Read the model definition and answer for the solid it produces. Units are mm, in the model's axes. Face numbers are marked on the shaded views. A direction names the side the tool comes from. Give positions to 0.01 mm unless a question says otherwise; leave off trailing zeros. Loops run counter-clockwise (first coordinate to the right, second up) from the corner with the lowest first, then second, coordinate; pieces in that order, holes last.
(1) Find section B-B, the plane y = 15. Write down the section's boundary in (x, z).
(2) Which of the six approach directions +Z, -Z, +X, -X, +Y, -Y give full straight-line access (tool end or side, diameter ignored) to the marked faces 4, 5 and 6?
(3) Find section D-D, the plane x = -5. Write down the section's boundary in (y, z), then the cut area to 3 significant figures.
(4) Determine the mould class of the marked faces 1, 2 and 3 for opening direction X: pulls with the +X half, pulls with the -X half, needs draft (parallel to the pull), parting line crosses it, or undercut.
(5) Find section C-C, the plane z = 1.5. Write down the section's boundary in (x, y).
(6) Each of these flat-tipped pins is pushed along its axis until it touches: P1, Ø4.5, axis at x = 7.5, y = 15, coming from the +Z side; P2, Ø4, axis at y = 10.5, z = 3, coming from the -X side; P3, Ø4, axis at x = -5, z = 6, coming from the +Y side. Where does it stop, or does it pass through?
(7) Find section A-A, the plane x = 7.5. Write down the section's boundary in (y, z), then the cut area to 3 significant figures.
(8) Straight lines are drawn through the part: probe 1 along Y at (x, z) = (7.5, 2.5); probe 2 along X at (y, z) = (0.7, 0); probe 3 along Z at (x, y) = (-5, 4.1). For each, find the intervals that lie inside material, in ascending order.
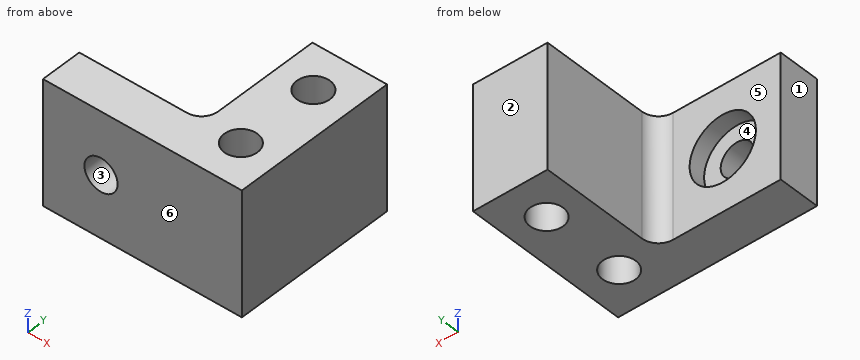
```python
from build123d import *

# Parameters (mm, degrees)
SKETCH1_W           = 24
SKETCH1_H           = 15
BOSS_EXTRUDE2_DEPTH = 5
SKETCH8_W           = 9
SKETCH8_H           = 15
BOSS_EXTRUDE3_DEPTH = 15
CUT_EXTRUDE3_REACH  = 7
SKETCH10_R          = 2
SKETCH9_R           = 4
CUT_EXTRUDE4_DEPTH  = 2
CUT_EXTRUDE5_REACH  = 17
SKETCH11_R          = 2
FILLET4_R           = 2


with BuildPart() as part:
    # Sketch1 → Boss-Extrude2 (new body)
    with BuildSketch(Plane(origin=(0, 0, 0), x_dir=(1, 0, 0), z_dir=(0, 1, 0))):
        Rectangle(SKETCH1_W, SKETCH1_H)
    extrude(amount=BOSS_EXTRUDE2_DEPTH)

    # Sketch8 → Boss-Extrude3 (add)
    with BuildSketch(Plane(origin=(0, 5, 0), x_dir=(1, 0, 0), z_dir=(0, 1, 0))):
        with Locations((7.5, 0)):
            Rectangle(SKETCH8_W, SKETCH8_H)
    extrude(amount=BOSS_EXTRUDE3_DEPTH)

    # Sketch10 → Cut-Extrude3 (cut, up to next)
    with BuildSketch(Plane(origin=(0, 5, 0), x_dir=(1, 0, 0), z_dir=(0, 1, 0)), mode=Mode.PRIVATE) as cut_extrude3_sk1:
        with Locations((-5, 0)):
            Circle(SKETCH10_R)
    cut_extrude3_tool1 = extrude(cut_extrude3_sk1.sketch, amount=-CUT_EXTRUDE3_REACH, mode=Mode.PRIVATE) & part.part
    add(cut_extrude3_tool1.solids().sort_by_distance((-5, 5, 0))[0], mode=Mode.SUBTRACT)

    # Sketch9 → Cut-Extrude4 (cut)
    with BuildSketch(Plane(origin=(0, 5, 0), x_dir=(1, 0, 0), z_dir=(0, 1, 0))):
        with Locations((-5, 0)):
            Circle(SKETCH9_R)
    extrude(amount=-CUT_EXTRUDE4_DEPTH, mode=Mode.SUBTRACT)

    # Sketch11 → Cut-Extrude5 (cut, up to next)
    with BuildSketch(Plane.XY.offset(7.5), mode=Mode.PRIVATE) as cut_extrude5_sk1:
        with Locations((7.5, 15)):
            Circle(SKETCH11_R)
    cut_extrude5_tool1 = extrude(cut_extrude5_sk1.sketch, amount=-CUT_EXTRUDE5_REACH, mode=Mode.PRIVATE) & part.part
    add(cut_extrude5_tool1.solids().sort_by_distance((7.5, 15, 7.5))[0], mode=Mode.SUBTRACT)
    # Sketch11 → Cut-Extrude5 (cut, up to next)
    with BuildSketch(Plane.XY.offset(7.5), mode=Mode.PRIVATE) as cut_extrude5_sk2:
        with Locations((7.5, 5)):
            Circle(SKETCH11_R)
    cut_extrude5_tool2 = extrude(cut_extrude5_sk2.sketch, amount=-CUT_EXTRUDE5_REACH, mode=Mode.PRIVATE) & part.part
    add(cut_extrude5_tool2.solids().sort_by_distance((7.5, 5, 7.5))[0], mode=Mode.SUBTRACT)

    # Fillet4
    fillet4_edges = [part.edges().sort_by_distance(p)[0] for p in [
        (3, 5, 0),
    ]]
    fillet(fillet4_edges, radius=FILLET4_R)


solid = part.part
```
Entries:
1. outline: (3, -7.5) - (5.5, -7.5) - (5.5, 7.5) - (3, 7.5) - close; (9.5, -7.5) - (12, -7.5) - (12, 7.5) - (9.5, 7.5) - close
2. face 4: +Y
2. face 5: +Z, -Z, -X, +Y
2. face 6: +Z, -Z, +X, -X, -Y
3. outline: (0, -7.5) - (5, -7.5) - (5, -4) - (3, -4) - (3, -2) - (0, -2) - close; (0, 2) - (3, 2) - (3, 4) - (5, 4) - (5, 7.5) - (0, 7.5) - close
3. area: 47.0 mm2
4. face 1: pulls with the -X half
4. face 2: needs draft
4. face 3: undercut
5. outline: (-12, 0) - (-6.32, 0) - (-6.32, 3) - (-8.71, 3) - (-8.71, 5) - (-12, 5) - close; (-3.68, 0) - (12, 0) - (12, 20) - (3, 20) - (3, 7) arc R2 cw to (1, 5) - (-1.29, 5) - (-1.29, 3) - (-3.68, 3) - close; hole circle Ø4 at (7.5, 5); hole circle Ø4 at (7.5, 15)
6. P1: stops at z = 7.5
6. P2: stops at x = 3
6. P3: stops at y = 5
7. outline: (0, -7.5) - (3, -7.5) - (3, 7.5) - (0, 7.5) - close; (7, -7.5) - (13, -7.5) - (13, 7.5) - (7, 7.5) - close; (17, -7.5) - (20, -7.5) - (20, 7.5) - (17, 7.5) - close
7. area: 180 mm2
8. probe 1: y = 0 to 3, 7 to 13, 17 to 20
8. probe 2: x = -12 to -7, -3 to 12
8. probe 3: z = -7.5 to -4, 4 to 7.5
